For this review, take the finished solid that the model builds, in its own axes (mm). Face numbers are marked on the shaded views. Coordinates: 2 decimals unless noted, no trailing zeros. Loops run counter-clockwise (first coordinate to the right, second up) from the corner with the lowest first, then second, coordinate; pieces in that order, holes last.
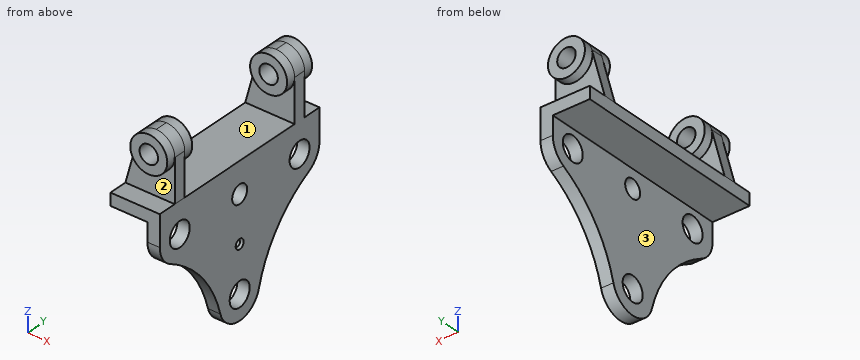
```python
from build123d import *
from build123d.topology import SkipClean

# Parameters (mm, degrees)
BASE_EXTRUDE_DEPTH                                = 6.35
SKETCH4_R                                         = 6.35
SKETCH4_R_2                                       = 4.7625
CUT_EXTRUDE1_DEPTH                                = 128.158650905
SKETCH3_W                                         = 25.4
SKETCH3_H                                         = 101.6
BOSS_EXTRUDE1_DEPTH                               = 6.35
BOSS_EXTRUDE2_DEPTH                               = 3.175
SKETCH6_R                                         = 9.525
BOSS_EXTRUDE3_DEPTH                               = 7.9375
SKETCH7_R                                         = 4.7625
CUT_EXTRUDE2_DEPTH                                = 125.686983708
CSK_FOR_3_FLAT_HEAD_MACHINE_SCREW_100_D           = 2.794
CSK_FOR_3_FLAT_HEAD_MACHINE_SCREW_100_DEPTH       = 4.7625
CSK_FOR_3_FLAT_HEAD_MACHINE_SCREW_100_CSINK_D     = 5.0546
CSK_FOR_3_FLAT_HEAD_MACHINE_SCREW_100_CSINK_ANGLE = 100
CSK_FOR_3_FLAT_HEAD_MACHINE_SCREW_100_TIP         = 0.839402285


with BuildPart() as part:
    # Sketch2 → Base-Extrude (new body)
    with BuildSketch(Plane(origin=(0, 0, 0), x_dir=(0, 0, -1), z_dir=(1, 0, 0))):
        with BuildLine():
            Line((0, 0), (0, 101.6))
            Line((0, 101.6), (15.875, 101.6))
            ThreePointArc((15.875, 101.6), (22.439736017, 99.771717483), (27.114363043, 94.813266304))
            ThreePointArc((27.114363043, 94.813266304), (43.64304274, 74.794428425), (66.801863043, 63.063266304))
            ThreePointArc((66.801863043, 63.063266304), (76.2, 50.8), (66.801863043, 38.536733696))
            ThreePointArc((66.801863043, 38.536733696), (43.64304274, 26.805571575), (27.114363043, 6.786733696))
            ThreePointArc((27.114363043, 6.786733696), (22.439736017, 1.828282517), (15.875, 0))
            Line((15.875, 0), (0, 0))
        make_face()
    extrude(amount=BASE_EXTRUDE_DEPTH)

    # Sketch4 → Cut-Extrude1 (cut, through all)
    with BuildSketch(Plane(origin=(6.35, 0, 0), x_dir=(0, 0, -1), z_dir=(1, 0, 0))):
        with Locations((63.5, 50.8)):
            Circle(SKETCH4_R)
        with Locations((15.875, 88.9)):
            Circle(SKETCH4_R)
        with Locations((15.875, 12.7)):
            Circle(SKETCH4_R)
        with Locations((15.875, 50.8)):
            Circle(SKETCH4_R_2)
    extrude(amount=-CUT_EXTRUDE1_DEPTH, mode=Mode.SUBTRACT)

    # Sketch3 → Boss-Extrude1 (add)
    with BuildSketch(Plane.XY):
        with Locations((-6.35, 50.8)):
            Rectangle(SKETCH3_W, SKETCH3_H)
    extrude(amount=-BOSS_EXTRUDE1_DEPTH)

    # Sketch5 → Boss-Extrude2 (add, symmetric)
    with BuildSketch(Plane(origin=(0, 88.9, 0), x_dir=(-1, 0, 0), z_dir=(0, 1, 0))):
        with BuildLine():
            Line((19.05, 0), (-6.35, 0))
            Line((-6.35, 0), (-6.35, 22.225))
            ThreePointArc((-6.35, 22.225), (1.921253552, 31.667126076), (12.369946424, 24.710676017))
            Line((12.369946424, 24.710676017), (19.05, 0))
        make_face()
    boss_extrude2 = extrude(amount=BOSS_EXTRUDE2_DEPTH, both=True)

    # Sketch6 → Boss-Extrude3 (add, symmetric)
    with SkipClean():  # the faces are left unmerged after this step: merging them gives an invalid solid
        with BuildSketch(Plane(origin=(0, 88.9, 0), x_dir=(-1, 0, 0), z_dir=(0, 1, 0))):
            with Locations(Location((3.175, 22.225, 0), (0, 0, 90))):
                Circle(SKETCH6_R)
        boss_extrude3 = extrude(amount=BOSS_EXTRUDE3_DEPTH, both=True)

    # Sketch7 → Cut-Extrude2 (cut, through all)
    with SkipClean():  # the faces are left unmerged after this step: merging them gives an invalid solid
        with BuildSketch(Plane(origin=(0, 96.8375, 0), x_dir=(-1, 0, 0), z_dir=(0, 1, 0))):
            with Locations(Location((3.175, 22.225, 0), (0, 0, 90))):
                Circle(SKETCH7_R)
        cut_extrude2 = extrude(amount=-CUT_EXTRUDE2_DEPTH, mode=Mode.SUBTRACT)

    # Mirror2: Boss-Extrude2, Boss-Extrude3, Cut-Extrude2 across plane
    with SkipClean():  # the faces are left unmerged after this step: merging them gives an invalid solid
        add(boss_extrude2.mirror(Plane.ZX.offset(50.8)))
        add(boss_extrude3.mirror(Plane.ZX.offset(50.8)))
        add(cut_extrude2.mirror(Plane.ZX.offset(50.8)), mode=Mode.SUBTRACT)

    # CSK for #3 Flat Head Machine Screw (100)1
    with Locations(Plane(origin=(6.35, 0, 0), x_dir=(0, 0, -1), z_dir=(1, 0, 0))):
        with Locations((39.6875, 50.8)):
            CounterSinkHole(CSK_FOR_3_FLAT_HEAD_MACHINE_SCREW_100_D / 2, CSK_FOR_3_FLAT_HEAD_MACHINE_SCREW_100_CSINK_D / 2, depth=CSK_FOR_3_FLAT_HEAD_MACHINE_SCREW_100_DEPTH, counter_sink_angle=CSK_FOR_3_FLAT_HEAD_MACHINE_SCREW_100_CSINK_ANGLE)
            with Locations((0, 0, -(CSK_FOR_3_FLAT_HEAD_MACHINE_SCREW_100_DEPTH + CSK_FOR_3_FLAT_HEAD_MACHINE_SCREW_100_TIP / 2))):  # 118° drill point
                Cone(0, CSK_FOR_3_FLAT_HEAD_MACHINE_SCREW_100_D / 2, CSK_FOR_3_FLAT_HEAD_MACHINE_SCREW_100_TIP, mode=Mode.SUBTRACT)


solid = part.part
```
Q1. The part is to be moulded in two halves that separate along Y. For the marked faces 1, 2 and 3, say which applies: +Y half, -Y half, draft (parallel to the pull), parting line (faces both ways), or undercut.
Q2. Consider section A-A (y = 14.5). Count the separate pieces of the cut face and the enclosed holes in it, then the cut area to 3 significant figures.
Q3. For pin 1 Ø1.5 at (x, y) = (-7, 77) entering from -Z; pin 2 Ø1.5 at (x, z) = (-12, 19.5) entering from -Y; pin 3 Ø9.5 at (x, z) = (-5, 23.5) entering from +Y; pin 4 Ø5.5 at (x, z) = (-4.5, 21.5) entering from +Y, all flat-tipped, find the tip position at first contact; note any pin that passes through.
Q4. Consider section B-B (z = -63.5). State the section outline as (x, y) points.
Q5. Wall thickness on probe 1 along Y at (x, z) = (-0.25, 8) (3 decimals); probe 2 along Y at (x, z) = (2.5, -20); probe 3 along Y at (x, z) = (1, 25): over which ranges is each line inside the solid? List them lowest first.
Q6. Consider section C-C (z = -14.5). State the section outline as (x, y) points, then the cut area to 3 significant figures.
Model answer:
1. face 1: undercut
1. face 2: -Y half
1. face 3: draft
2. separate pieces: 2
2. enclosed holes: 1
2. area: 816 mm2
3. pin 1: stops at z = -6.35
3. pin 2: stops at y = 4.76
3. pin 3: stops at y = 96.84
3. pin 4: passes through
4. outline: (0, 37.55) - (6.35, 37.55) - (6.35, 44.45) - (0, 44.45) - close; (0, 57.15) - (6.35, 57.15) - (6.35, 64.05) - (0, 64.05) - close
5. probe 1: y = 9.525 to 15.875, 85.725 to 92.075
5. probe 2: y = 0.69 to 7.87, 17.53 to 48.42, 53.18 to 84.07, 93.73 to 100.91
5. probe 3: y = 4.76 to 20.64, 80.96 to 96.84
6. outline: (0, 0) - (6.35, 0) - (6.35, 6.5) - (0, 6.5) - close; (0, 18.9) - (6.35, 18.9) - (6.35, 46.24) - (0, 46.24) - close; (0, 55.36) - (6.35, 55.36) - (6.35, 82.7) - (0, 82.7) - close; (0, 95.1) - (6.35, 95.1) - (6.35, 101.6) - (0, 101.6) - close
6. area: 430 mm2
